```python
from build123d import *

# Parameters (mm, degrees)
SKETCH_2_R      = 1
EXTRUDE_1_DEPTH = 2
EXTRUDE_2_DEPTH = 2
EXTRUDE_3_DEPTH = 2.8
SKETCH_5_R      = 1.75
EXTRUDE_4_DEPTH = 4.8
EXTRUDE_START   = 1.2
SKETCH_6_R      = 1.75
EXTRUDE_5_DEPTH = 1.2
FILLET_1_R      = 1


with BuildPart() as part:
    # 草图2 → 凸台-拉伸1 (new body)
    with BuildSketch(Plane(origin=(0, 0, -1.538354077), x_dir=(-1, 0, 0), z_dir=(0, 0, -1))):
        with BuildLine():
            Line((-22.942959106, -124.662212149), (-17.134907671, 121.132350923))
            ThreePointArc((-17.134907671, 121.132350923), (-16.793190136, 121.861742775), (-16.024570953, 122.102591063))
            ThreePointArc((-16.024570953, 122.102591063), (-14.009380987, 122.790837638), (-13.255665128, 124.782466708))
            ThreePointArc((-13.255665128, 124.782466708), (-12.992914403, 125.539491489), (-12.25871858, 125.860553721))
            Line((-12.25871858, 125.860553721), (12.25871858, 125.860553721))
            ThreePointArc((12.25871858, 125.860553721), (12.992914403, 125.539491489), (13.255665128, 124.782466708))
            ThreePointArc((13.255665128, 124.782466708), (14.009380087, 122.79083851), (16.024568463, 122.102590786))
            ThreePointArc((16.024568463, 122.102590786), (16.793187022, 121.861742062), (17.134904184, 121.13235055))
            Line((17.134904184, 121.13235055), (22.942959106, -124.662212156))
            Line((22.942959106, -124.662212156), (22.942959106, -124.904555532))
            ThreePointArc((22.942959106, -124.904555532), (22.626864313, -125.634126411), (21.878411771, -125.902470178))
            ThreePointArc((21.878411771, -125.902470178), (19.586380534, -127.089481736), (19.565603095, -129.670561341))
            Line((19.565603095, -129.670561341), (19.265011022, -129.670561341))
            Line((19.265011022, -129.670561341), (19.265011022, -130.670561341))
            Line((19.265011022, -130.670561341), (23.942959106, -130.670561341))
            Line((23.942959106, -130.670561341), (23.942959106, -124.650398948))
            Line((23.942959106, -124.650398948), (18.052063488, 124.649948906))
            Line((18.052063488, 124.649948906), (18.052059944, 126.860553721))
            Line((18.052059944, 126.860553721), (-18.052059944, 126.860553721))
            Line((-18.052059944, 126.860553721), (-18.052059944, 124.65024892))
            Line((-18.052059944, 124.65024892), (-23.942959106, -124.650398948))
            Line((-23.942959106, -124.650398948), (-23.942959106, -130.670561341))
            Line((-23.942959106, -130.670561341), (-19.234988978, -130.670561341))
            Line((-19.234988978, -130.670561341), (-19.234988978, -129.670561341))
            Line((-19.234988978, -129.670561341), (-19.646017972, -129.670561341))
            ThreePointArc((-19.646017972, -129.670561341), (-19.548027097, -127.027128176), (-21.878411771, -125.775469924))
            ThreePointArc((-21.878411771, -125.775469924), (-22.626864313, -125.507126157), (-22.942959106, -124.777555278))
            Line((-22.942959106, -124.777555278), (-22.942959106, -124.662212149))
        make_face()
        with Locations((-21.717043434, -128.270256541)):
            Circle(SKETCH_2_R, mode=Mode.SUBTRACT)
        with Locations((21.717043434, -128.397256794)):
            Circle(SKETCH_2_R, mode=Mode.SUBTRACT)
        with Locations((-15.748031496, 124.587249174)):
            Circle(SKETCH_2_R, mode=Mode.SUBTRACT)
        with Locations((15.748031496, 124.587249174)):
            Circle(SKETCH_2_R, mode=Mode.SUBTRACT)
    extrude(amount=EXTRUDE_1_DEPTH)

    # 草图3 → 凸台-拉伸2 (add)
    with BuildSketch(Plane(origin=(0, 0, -3.538354077), x_dir=(-1, 0, 0), z_dir=(0, 0, -1))):
        Polygon((26.942959106, -124.614959326), (21.052063431, 124.685390934), (21.052055134, 129.860553721), (-21.052059944, 129.860553721), (-21.052059944, 124.685688522), (-26.942959106, -124.614959347), (-26.942959106, -133.670561341), (26.942959106, -133.670561341), align=None)
        Polygon((18.052059944, 126.860553721), (-18.052059944, 126.860553721), (-18.052059944, 124.65024892), (-23.942959106, -124.650398948), (-23.942959106, -130.670561341), (23.942959106, -130.670561341), (23.942959106, -124.650398948), (18.052063488, 124.649948906), align=None, mode=Mode.SUBTRACT)
    extrude(amount=-EXTRUDE_2_DEPTH)

    # 草图4 → 凸台-拉伸3 (add)
    with BuildSketch(Plane.XY.offset(-1.538354077)):
        Polygon((-21.052063431, 124.685390934), (-26.942959106, -124.614959326), (-26.942959106, -133.670561341), (26.942959106, -133.670561341), (26.942959106, -124.614959347), (21.052059944, 124.685688522), (21.052059944, 129.860553721), (-21.052055134, 129.860553721), align=None)
        Polygon((-18.302059543, 127.110553721), (-18.302063484, 124.652902409), (-24.192959106, -124.647445647), (-24.192959106, -130.920561341), (24.192959106, -130.920561341), (24.192959106, -124.647445648), (18.302059944, 124.653202221), (18.302059944, 127.110553721), align=None, mode=Mode.SUBTRACT)
    extrude(amount=EXTRUDE_3_DEPTH)

    # 草图5 → 凸台-拉伸4 (add)
    # profile 1 of 2: a face of its own
    with BuildSketch(Plane.XY.offset(1.261645923)):
        Polygon((-26.942959106, -133.670561341), (26.942959106, -133.670561341), (26.942959106, -138.670561341), (26.942959106, -141.170561341), (-26.942959106, -141.170561341), (-26.942959106, -138.670561341), align=None)
        with Locations((2.405e-06, -136.170561341)):
            Circle(SKETCH_5_R, mode=Mode.SUBTRACT)
        with Locations((21.942959106, -136.170561341)):
            Circle(SKETCH_5_R, mode=Mode.SUBTRACT)
        with Locations((-21.942959106, -136.170561341)):
            Circle(SKETCH_5_R, mode=Mode.SUBTRACT)
    # profile 2 of 2: a face of its own
    with BuildSketch(Plane.XY.offset(1.261645923)):
        Polygon((21.052059944, 129.860553721), (-21.052055134, 129.860553721), (-21.052055134, 134.860553721), (-21.052055134, 137.360553721), (21.052059944, 137.360553721), (21.052059944, 134.860553721), align=None)
        with Locations((-17.052055134, 132.360553721)):
            Circle(SKETCH_5_R, mode=Mode.SUBTRACT)
        with Locations((17.052059944, 132.360553721)):
            Circle(SKETCH_5_R, mode=Mode.SUBTRACT)
        with Locations((2.405e-06, 132.360553721)):
            Circle(SKETCH_5_R, mode=Mode.SUBTRACT)
    extrude(amount=-EXTRUDE_4_DEPTH)

    # 草图6 → 凸台-拉伸5 (add)
    # profile 1 of 2: a face of its own
    with BuildSketch(Plane.XY.offset(1.261645923).offset(EXTRUDE_START)):
        with BuildLine():
            Line((-26.942959106, -138.670561341), (-26.942959106, -141.170561341))
            Line((-26.942959106, -141.170561341), (26.942959106, -141.170561341))
            Line((26.942959106, -141.170561341), (26.942959106, -138.670561341))
            Line((26.942959106, -138.670561341), (26.942959106, -135.670561341))
            ThreePointArc((26.942959106, -135.670561341), (26.357172668, -134.256347779), (24.942959106, -133.670561341))
            Line((24.942959106, -133.670561341), (-24.942959106, -133.670561341))
            ThreePointArc((-24.942959106, -133.670561341), (-26.357172668, -134.256347779), (-26.942959106, -135.670561341))
            Line((-26.942959106, -135.670561341), (-26.942959106, -138.670561341))
        make_face()
        with Locations((21.942959106, -136.170561341)):
            Circle(SKETCH_6_R, mode=Mode.SUBTRACT)
        with Locations((2.405e-06, -136.170561341)):
            Circle(SKETCH_6_R, mode=Mode.SUBTRACT)
        with Locations((-21.942959106, -136.170561341)):
            Circle(SKETCH_6_R, mode=Mode.SUBTRACT)
    # profile 2 of 2: a face of its own
    with BuildSketch(Plane.XY.offset(1.261645923).offset(EXTRUDE_START)):
        with BuildLine():
            Line((21.052059944, 131.860553721), (21.052059944, 134.860553721))
            Line((21.052059944, 134.860553721), (21.052059944, 137.360553721))
            Line((21.052059944, 137.360553721), (-21.052055134, 137.360553721))
            Line((-21.052055134, 137.360553721), (-21.052055134, 134.860553721))
            Line((-21.052055134, 134.860553721), (-21.052055134, 131.860553721))
            ThreePointArc((-21.052055134, 131.860553721), (-20.466268697, 130.446340159), (-19.052055134, 129.860553721))
            Line((-19.052055134, 129.860553721), (19.052059944, 129.860553721))
            ThreePointArc((19.052059944, 129.860553721), (20.466273506, 130.446340159), (21.052059944, 131.860553721))
        make_face()
        with Locations((17.052059944, 132.360553721)):
            Circle(SKETCH_6_R, mode=Mode.SUBTRACT)
        with Locations((2.405e-06, 132.360553721)):
            Circle(SKETCH_6_R, mode=Mode.SUBTRACT)
        with Locations((-17.052055134, 132.360553721)):
            Circle(SKETCH_6_R, mode=Mode.SUBTRACT)
    extrude(amount=-EXTRUDE_5_DEPTH)

    # 圆角1
    # the kernel refuses this fillet: 1 mm, written as the material it adds along each edge
    with BuildSketch(Plane(origin=(24.942959106, -135.670561341, 1.261645923), x_dir=(0.31484580408697693, -0.9491428341660831, 0), z_dir=(-0.9491428341660831, -0.31484580408697693, 0))) as fillet_1_piece_1_section:
        with BuildLine():
            CenterArc((2 + FILLET_1_R, FILLET_1_R), FILLET_1_R, 180, 90)
            Line((2, FILLET_1_R), (2, 0))
            Line((2, 0), (2 + FILLET_1_R, 0))
        make_face()
    fillet_1_piece_1 = revolve(axis=Axis((24.942959106, -135.670561341, 1.261645923), (0, 0, 1)), revolution_arc=161.648494619, mode=Mode.PRIVATE)
    fillet_1_piece_1 = split(fillet_1_piece_1, bisect_by=Plane(origin=(26.942959106, -134.20836544, 1.533797611), z_dir=(-1, 0, 0)), keep=Keep.TOP, mode=Mode.PRIVATE)
    add(fillet_1_piece_1)
    with BuildSketch(Plane(origin=(-24.942959106, -135.670561341, 1.261645923), x_dir=(0, 1, 0), z_dir=(1, 0, 0))) as fillet_1_piece_2_section:
        with BuildLine():
            CenterArc((2 + FILLET_1_R, FILLET_1_R), FILLET_1_R, 180, 90)
            Line((2 + FILLET_1_R, 0), (2, 0))
            Line((2, 0), (2, FILLET_1_R))
        make_face()
    fillet_1_piece_2 = revolve(axis=Axis((-24.942959106, -135.670561341, 1.261645923), (0, 0, 1)), revolution_arc=161.648494619, mode=Mode.PRIVATE)
    fillet_1_piece_2 = split(fillet_1_piece_2, bisect_by=Plane(origin=(-26.942959106, -134.20836489, 1.533796612), z_dir=(1, 0, 0)), keep=Keep.TOP, mode=Mode.PRIVATE)
    add(fillet_1_piece_2)
    with BuildSketch(Plane(origin=(-19.052055134, 131.860553721, 1.261645923), x_dir=(-0.31484580408698715, 0.9491428341660799, 0), z_dir=(0.9491428341660799, 0.31484580408698715, 0))) as fillet_1_piece_3_section:
        with BuildLine():
            CenterArc((2 + FILLET_1_R, FILLET_1_R), FILLET_1_R, 180, 90)
            Line((2, FILLET_1_R), (2, 0))
            Line((2, 0), (2 + FILLET_1_R, 0))
        make_face()
    fillet_1_piece_3 = revolve(axis=Axis((-19.052055134, 131.860553721, 1.261645923), (0, 0, 1)), revolution_arc=161.648494619, mode=Mode.PRIVATE)
    fillet_1_piece_3 = split(fillet_1_piece_3, bisect_by=Plane(origin=(-21.052055134, 130.742519817, 1.42831269), z_dir=(1, 0, 0)), keep=Keep.TOP, mode=Mode.PRIVATE)
    add(fillet_1_piece_3)
    with BuildSketch(Plane(origin=(19.052059944, 131.860553721, 1.261645923), x_dir=(0, -1, 0), z_dir=(-1, 0, 0))) as fillet_1_piece_4_section:
        with BuildLine():
            CenterArc((2 + FILLET_1_R, FILLET_1_R), FILLET_1_R, 180, 90)
            Line((2, FILLET_1_R), (2, 0))
            Line((2, 0), (2 + FILLET_1_R, 0))
        make_face()
    fillet_1_piece_4 = revolve(axis=Axis((19.052059944, 131.860553721, 1.261645923), (0, 0, 1)), revolution_arc=161.648494619, mode=Mode.PRIVATE)
    fillet_1_piece_4 = split(fillet_1_piece_4, bisect_by=Plane(origin=(21.052059944, 129.648450881, 1.424284575), z_dir=(-1, 0, 0)), keep=Keep.TOP, mode=Mode.PRIVATE)
    add(fillet_1_piece_4)
    with BuildSketch(Plane(origin=(24.942959106, -133.670561341, 1.261645923), x_dir=(0, 1, 0), z_dir=(-1, 0, 0))) as fillet_1_piece_5:
        with BuildLine():
            CenterArc((FILLET_1_R, -FILLET_1_R), FILLET_1_R, 90, 90)
            Line((0, -FILLET_1_R), (0, 0))
            Line((0, 0), (FILLET_1_R, 0))
        make_face()
    extrude(amount=49.885918212)
    with BuildSketch(Plane(origin=(-19.052055134, 129.860553721, 1.261645923), x_dir=(0, -1, 0), z_dir=(1, 0, 0))) as fillet_1_piece_6:
        with BuildLine():
            CenterArc((FILLET_1_R, -FILLET_1_R), FILLET_1_R, 90, 90)
            Line((0, -FILLET_1_R), (0, 0))
            Line((0, 0), (FILLET_1_R, 0))
        make_face()
    extrude(amount=38.104115079)


solid = part.part
```
Can you work these out from the model? Positions are in its coordinate system, mm. A direction names the side the tool comes from. Coordinates: 2 decimals unless noted, no trailing zeros. Loops run counter-clockwise (first coordinate to the right, second up) from the corner with the lowest first, then second, coordinate; pieces in that order, holes last.
Item 1: Suppose I cut it at B-B (y = 72). Please give me the cut outline in (x, z), then the cut area to 3 significant figures.
Answers below:
outline: (-22.3, -3.54) - (-18.3, -3.54) - (-18.3, -1.54) - (-19.55, -1.54) - (-19.55, 1.26) - (-22.3, 1.26) - close; (18.3, -3.54) - (22.3, -3.54) - (22.3, 1.26) - (19.55, 1.26) - (19.55, -1.54) - (18.3, -1.54) - close
area: 31.4 mm2
Item 2: Suppose I cut it at A-A (x = 7). Please give me the cut outline in (y, z), then the cut area to 3 significant figures.
Answers below:
outline: (-141.17, -3.54) - (-130.67, -3.54) - (-130.67, -1.54) - (-130.92, -1.54) - (-130.92, 1.26) - (-132.67, 1.26) arc R1 cw to (-133.67, 2.26) - (-133.67, 2.46) - (-141.17, 2.46) - close; (125.86, -3.54) - (137.36, -3.54) - (137.36, 2.46) - (129.86, 2.46) - (129.86, 2.26) arc R1 cw to (128.86, 1.26) - (127.11, 1.26) - (127.11, -1.54) - (125.86, -1.54) - close
area: 120 mm2
Item 3: Please list where these lines run through material, in increasing order: L1, parallel to Y at x = -10.5, z = -0.25; L2, parallel to Y at x = -7.5, z = -2.5; L3, parallel to X at y = 44, z = -0.5.
Answers below:
L1: y = -141.17 to -130.92, 127.11 to 137.36
L2: y = -141.17 to -130.67, 125.86 to 137.36
L3: x = -22.96 to -20.21, 20.21 to 22.96
Item 4: Which directions (+Z, -Z, +X, -X, +Y, -Y) give clear straight access to the entire face, cutting with the end or side of a thin tool? Please do faces 1 (the face through (20, 8, -1.538)), 2 (the face through (21.052, 131, 0)), 3 (the face through (-26.943, -133, -1)).
Answers below:
face 1: +Z
face 2: +Z, -Z, +X, +Y
face 3: +Z, -Z, -X, +Y, -Y
Item 5: If we mould it in two halves opening along Y, with no side actions, what happens to faces 4 (the face through (-0.4, -138.2, 2.462)), 5 (the face through (-22, -11, 1.262)), 6 (the face through (0, 137.361, 0))? For each: released by +Y, released by -Y, zero draft, split by the parting line, or undercut.
Answers below:
face 4: zero draft
face 5: undercut
face 6: released by +Y
Item 6: I'm going to push flat-ended pins straight in: pin 1 (3 mm diameter, centred on y = 132.5, z = -2, fed in from +X); pin 2 (4.5 mm diameter, centred on x = 21.94, y = -136.17, fed in from -Z); pin 3 (1.4 mm diameter, centred on y = 127, z = -2, fed in from -X); pin 4 (1.5 mm diameter, centred on y = -70.5, z = -3, fed in from +X). Where does each tip first touch, or does it pass through?
Answers below:
pin 1: stops at x = 21.05
pin 2: stops at z = -3.54
pin 3: stops at x = -21.05
pin 4: stops at x = 25.68
Item 7: Suppose I cut it at C-C (z = 0). Please give me the cut outline in (x, y), then the cut area to 3 significant figures.
Answers below:
outline: (-26.94, -141.17) - (26.94, -141.17) - (26.94, -124.61) - (21.05, 124.69) - (21.05, 137.36) - (-21.05, 137.36) - (-21.05, 129.86) - (-21.05, 124.69) - (-26.94, -124.61) - close; hole (-24.19, -130.92) - (24.19, -130.92) - (24.19, -124.65) - (18.3, 124.65) - (18.3, 127.11) - (-18.3, 127.11) - (-18.3, 124.65) - (-24.19, -124.65) - close; hole circle Ø3.5 at (-21.94, -136.17); hole circle Ø3.5 at (-17.05, 132.36); hole circle Ø3.5 at (0, -136.17); hole circle Ø3.5 at (0, 132.36); hole circle Ø3.5 at (17.05, 132.36); hole circle Ø3.5 at (21.94, -136.17)
area: 2,350 mm2
